```python
from build123d import *

# Parameters (mm, degrees)
ESQUISSE1_W        = 30.5
ESQUISSE1_H        = 25
BOSS_EXTRU_1_DEPTH = 1
BOSS_EXTRU_2_DEPTH = 1
ESQUISSE3_R        = 2.5
BOSS_EXTRU_3_DEPTH = 23
ESQUISSE4_R        = 4
BOSS_EXTRU_4_DEPTH = 18


with BuildPart() as part:
    # Esquisse1 → Boss.-Extru.1 (new body)
    with BuildSketch(Plane(origin=(0, 0, 0), x_dir=(1, 0, 0), z_dir=(0, 1, 0))):
        Rectangle(ESQUISSE1_W, ESQUISSE1_H)
    extrude(amount=BOSS_EXTRU_1_DEPTH)

    # Esquisse2 → Boss.-Extru.2 (add)
    with BuildSketch(Plane.XY.offset(12.5)):
        Polygon((15.199854564, 1.034402705), (15.467639278, -21.965597295), (13.467639278, -21.965597295), (-4.785365363, -3.659095072), (-15.23307626, -3.659095072), (-15.25, 1), align=None)
    boss_extru_2 = extrude(amount=-BOSS_EXTRU_2_DEPTH)

    # Symétrie1: Boss.-Extru.2 across plane
    add(boss_extru_2.mirror(Plane.XY))

    # Esquisse3 → Boss.-Extru.3 (add)
    with BuildSketch(Plane.XY.offset(-11.5)):
        with Locations(Location((14.132711903, -20.613073056, 0), (0, 0, 169.692708603))):
            Circle(ESQUISSE3_R)
    extrude(amount=BOSS_EXTRU_3_DEPTH)

    # Esquisse4 → Boss.-Extru.4 (add)
    with BuildSketch(Plane(origin=(0, 1, 0), x_dir=(1, 0, 0), z_dir=(0, 1, 0))):
        with Locations(Location((-4.931252749, 0, 0), (0, 0, 270))):
            Circle(ESQUISSE4_R)
    extrude(amount=BOSS_EXTRU_4_DEPTH)


solid = part.part
```
Part model, mm, in its own coordinate system. A direction names the side the tool comes from. Round coordinates to 2 decimals unless told otherwise and drop trailing zeros. Loops run counter-clockwise (first coordinate to the right, second up) from the corner with the lowest first, then second, coordinate; pieces in that order, holes last.
1. 3-axis set-ups, long thin cutter, end or side, ignore diameter. For faces 4 (the face through (14, -21.966, -12)), 5 (the face through (-0.965, 9.874, -0.521)), 6 (the face through (-10, -3.659, 12)): which of +Z, -Z, +X, -X, +Y, -Y reach the whole face in a straight line?
Solutions:
face 4: -Z, +X, -X, -Y
face 5: +Y
face 6: +Z, -Z, -X, -Y
2. Slice it at A-A (z = -6.5). Give the cut face in (x, y).
Solutions:
outline: (-15.25, 0) - (15.25, 0) - (15.25, 1) - (-15.25, 1) - close; circle Ø5 at (14.13, -20.61)
3. Two-plate mould, pull along Z, no slides. Class faces 1 (the face through (15.103, -18.309, -0.161)), 2 (the face through (4, -8, -12.5)), 3 (the face through (14, -21.966, 12)): pulls with the +Z half, pulls with the -Z half, needs draft (parallel to the pull), parting line crosses it, or undercut.
Solutions:
face 1: undercut
face 2: pulls with the -Z half
face 3: needs draft
4. Drill centre lines: line 1 along Z through (x, y) = (7, -1.5); line 2 along Y through (x, z) = (8, -6.5); line 3 along Y through (x, z) = (15, -2.5). Where is each one in solid material? Low to high.
Solutions:
line 1: z = -12.5 to -11.5, 11.5 to 12.5
line 2: y = 0 to 1
line 3: y = -22.96 to -18.27, 0 to 1
5. Flat gauge pins, fed straight in: pin 1 (0.8 mm diameter, centred on x = -10.5, z = -12, fed in from -Y); pin 2 (0.8 mm diameter, centred on x = 14.5, z = -12, fed in from -Y); pin 3 (6 mm diameter, centred on x = -7.5, z = -0.5, fed in from -Y). Where does each tip first touch, or does it go through?
Solutions:
pin 1: stops at y = -3.66
pin 2: stops at y = -21.97
pin 3: stops at y = 0
6. Slice it at B-B (y = -2). Give the cut face in (x, z).
Solutions:
outline: (-15.24, -12.5) - (15.24, -12.5) - (15.24, -11.5) - (-15.24, -11.5) - close; (-15.24, 11.5) - (15.24, 11.5) - (15.24, 12.5) - (-15.24, 12.5) - close
